from build123d import *

# Parameters (mm, degrees)
F0_R     = 1.65
F0_R_2   = 6
F1_DEPTH = 2
F2_DEPTH = 0.5


with BuildPart() as f1:
    # F0 (on Top) → F1 (new body)
    with BuildSketch(Plane.XY):
        with BuildLine():
            Line((-3.731809, 13.94), (-7.930095, 3.06))
            ThreePointArc((-7.930095, 3.06), (-8.5, 0), (-7.930095, -3.06))
            Line((-7.930095, -3.06), (-3.731809, -13.94))
            ThreePointArc((-3.731809, -13.94), (0, -16.5), (3.731809, -13.94))
            Line((3.731809, -13.94), (7.930095, -3.06))
            ThreePointArc((7.930095, -3.06), (8.5, 0), (7.930095, 3.06))
            Line((7.930095, 3.06), (3.731809, 13.94))
            ThreePointArc((3.731809, 13.94), (0, 16.5), (-3.731809, 13.94))
        make_face()
        with Locations((0, -12.5)):
            Circle(F0_R, mode=Mode.SUBTRACT)
        Circle(F0_R_2, mode=Mode.SUBTRACT)
        with Locations((0, 12.5)):
            Circle(F0_R, mode=Mode.SUBTRACT)
    extrude(amount=F1_DEPTH)

    # F0 (on Top) → F2 (join)
    with BuildSketch(Plane.XY):
        Circle(F0_R_2)
    extrude(amount=F2_DEPTH)


solid = f1.part
Could you check a few things on this model? Use its own coordinates, in mm. A direction names the side the tool comes from. Give positions to 0.01 mm unless a question says otherwise; leave off trailing zeros. Order: outer loops, then holes, each group sorted by start corner. A loop starts at its lowest first (then second) coordinate and runs counter-clockwise, first axis right, second up. Notation, with made-up numbers: (12.25, 31.25) - (50.25, 31.25) arc R22 ccw to (50.25, 45.25) - close; hole circle Ø7 at (-17, 20.25). An arc over 180 degrees is marked (long way). Return JSON: item names as keys, results as strings. Group by question number.
Q1. Suppose I cut it at C-C, the plane y = 12.5. Please give me the cut outline in (x, z).
Q2. Which directions (+Z, -Z, +X, -X, +Y, -Y) give clear straight access to the entire face, cutting with the end or side of a thin tool? Please do faces 4 (the face through (8.5, 0, 1)), 5 (the face through (0, 0, 0.5)).
Q3. Please list where these lines run through material, in increasing order: line 1 along Y through (x, z) = (0, 1.15); line 2 along Y through (x, z) = (1.5, 1.85); line 3 along Z through (x, y) = (0.25, 1). Write a range as [from, to].
Q4. Will these pins go through, and if not, where does the flat tip stop? pin 1 Ø3 at (x, y) = (0, -12.5) entering from +Z; pin 2 Ø1 at (y, z) = (6, 0) entering from -X.
Q5. Thinking about a two-plate mould opening in Y: for faces 1 (the face through (6, -3, 2)), 2 (the face through (-8.5, 0, 1)), 3 (the face through (-6, 0, 1)), which applies, pulls with the +Y half, pulls with the -Y half, needs draft (parallel to the pull), parting line crosses it, or undercut?
Q6. Suppose I cut it at D-D, the plane y = -3.5. Please give me the cut outline in (x, z).
Q7. Suppose I cut it at B-B, the plane z = 1.05. Please give me the cut outline in (x, y).
Q8. Suppose I cut it at A-A, the plane x = 0. Please give me the cut outline in (y, z), and give its area (3 significant figures).
Resolved:
{
 "1": {"outline": "(-4.29, 0) - (-1.65, 0) - (-1.65, 2) - (-4.29, 2) - close; (1.65, 0) - (4.29, 0) - (4.29, 2) - (1.65, 2) - close"},
 "2": {"face 4": "+Z, -Z, +X", "face 5": "+Z"},
 "3": {"line 1": "y = [-16.5, -14.15], [-10.85, -6], [6, 10.85], [14.15, 16.5]", "line 2": "y = [-16.21, -13.19], [-11.81, -5.81], [5.81, 11.81], [13.19, 16.21]", "line 3": "z = [0, 0.5]"},
 "4": {"pin 1": "passes through", "pin 2": "stops at x = -6.99"},
 "5": {"face 1": "needs draft", "face 2": "parting line crosses it", "face 3": "undercut"},
 "6": {"outline": "(-7.76, 0) - (7.76, 0) - (7.76, 2) - (4.87, 2) - (4.87, 0.5) - (-4.87, 0.5) - (-4.87, 2) - (-7.76, 2) - close"},
 "7": {"outline": "(-7.93, -3.06) - (-3.73, -13.94) arc R4 ccw to (3.73, -13.94) - (7.93, -3.06) arc R8.5 ccw to (7.93, 3.06) - (3.73, 13.94) arc R4 ccw to (-3.73, 13.94) - (-7.93, 3.06) arc R8.5 ccw to start; hole circle Ø12 at (0, 0); hole circle Ø3.3 at (0, -12.5); hole circle Ø3.3 at (0, 12.5)"},
 "8": {"outline": "(-16.5, 0) - (-14.15, 0) - (-14.15, 2) - (-16.5, 2) - close; (-10.85, 0) - (10.85, 0) - (10.85, 2) - (6, 2) - (6, 0.5) - (-6, 0.5) - (-6, 2) - (-10.85, 2) - close; (14.15, 0) - (16.5, 0) - (16.5, 2) - (14.15, 2) - close", "area": "34.8 mm2"}
}
